Solid Edge part; units mm, degrees
sketch "Sketch1" plane through (0, 0, 0) normal (0, -1, 0) x (1, 0, 0)
  line L0 (25, -40) -> (25, 40)
  line L1 (25, 40) -> (-25, 40)
  line L2 (-25, 40) -> (-25, -40)
  line L3 (-25, -40) -> (25, -40)
  line L4 (22.5, -37.5) -> (22.5, 37.5)
  line L5 (22.5, 37.5) -> (-22.5, 37.5)
  line L6 (-22.5, 37.5) -> (-22.5, -37.5)
  line L7 (-22.5, -37.5) -> (22.5, -37.5)
extrude "Protrusion1" add sketch "Sketch1" against normal blind 35
sketch "Sketch2" plane through (0, 0, 0) normal (0, -1, 0) x (1, 0, 0)
  line L0 (22.5, 37.5) -> (-22.5, 37.5)
  line L1 (-22.5, 37.5) -> (-22.5, -37.5)
  line L2 (-22.5, -37.5) -> (22.5, -37.5)
  line L3 (22.5, -37.5) -> (22.5, 37.5)
extrude "ExtrudedProtrusion_2" add sketch "Sketch2" against normal blind 5
sketch "Sketch3" plane through (0, 0, 0) normal (0, -1, 0) x (0, 0, -1)
  circle A0 centre (-28.125, 11.25) radius 5
extrude "ExtrudedProtrusion_3" add sketch "Sketch3" along normal blind 3
pattern_linear "Pattern1" count 4 spacing 18.75 along (0, 0, -1) count 2 spacing 22.5 along (-1, 0, 0) of "ExtrudedProtrusion_3"
sketch "Sketch4" plane through (0, 5, 0) normal (0, 1, 0) x (0, 0, -1)
  line L0 (1, -9) -> (1, -22.5)
  line L1 (1, -22.5) -> (-1, -22.5)
  line L2 (-1, -22.5) -> (-1, -8.9443)
  line L3 (-1, -8.9443) -> (1, -9)
  line L4 (1, 9) -> (1, 22.5)
  line L5 (1, 22.5) -> (-1, 22.5)
  line L6 (-1, 22.5) -> (-1, 8.9443)
  line L7 (-1, 8.9443) -> (1, 9)
extrude "ExtrudedProtrusion_8" add sketch "Sketch4" along normal blind 20
sketch "Sketch5" plane through (0, 5, 19.25) normal (0, 1, 0) x (0, 0, 1)
  line L0 (-46.375, -22.5) -> (-48.375, -22.5)
  arc A0 (-48.375, -22.5) -> (-46.375, -22.5) centre (-47.375, -22.5) cw
extrude "ExtrudedProtrusion_9" add sketch "Sketch5" along normal blind 30
sketch "Sketch6" plane through (0, 5, -19.25) normal (0, 1, 0) x (1, 0, 0)
  line L0 (22.5, 8.875) -> (22.5, 9.875)
  line L1 (22.5, 7.875) -> (22.5, 8.875)
  arc A0 (22.5, 7.875) -> (22.5, 9.875) centre (22.5, 8.875) cw
  line L2 (22.5, -9.875) -> (22.5, -8.875)
  line L3 (22.5, -10.875) -> (22.5, -9.875)
  arc A1 (22.5, -10.875) -> (22.5, -8.875) centre (22.5, -9.875) cw
  line L4 (22.5, -28.625) -> (22.5, -27.625)
  line L5 (22.5, -29.625) -> (22.5, -28.625)
  arc A2 (22.5, -29.625) -> (22.5, -27.625) centre (22.5, -28.625) cw
  line L6 (22.5, -47.375) -> (22.5, -46.375)
  line L7 (22.5, -47.375) -> (22.5, -48.375)
  arc A3 (22.5, -48.375) -> (22.5, -46.375) centre (22.5, -47.375) cw
  line L8 (-22.5, -28.625) -> (-22.5, -29.625)
  line L9 (-22.5, -27.625) -> (-22.5, -28.625)
  arc A4 (-22.5, -27.625) -> (-22.5, -29.625) centre (-22.5, -28.625) cw
  line L10 (-22.5, -8.875) -> (-22.5, -10.875)
  arc A5 (-22.5, -8.875) -> (-22.5, -10.875) centre (-22.5, -9.875) cw
  line L11 (-22.5, -47.375) -> (-22.5, -48.375)
  line L12 (-22.5, -46.375) -> (-22.5, -47.375)
  arc A6 (-22.5, -46.375) -> (-22.5, -48.375) centre (-22.5, -47.375) cw
extrude "ExtrudedProtrusion_10" add sketch "Sketch6" along normal blind 30
sketch "Sketch7" plane through (0, 5, 0) normal (0, -1, 0) x (1, 0, 0)
  circle A0 centre (0, -25) radius 10
  circle A1 centre (0, -25) radius 7.5
  circle A2 centre (0, 0) radius 10
  circle A3 centre (0, 0) radius 7.5
  circle A4 centre (0, 25) radius 10
  circle A5 centre (0, 25) radius 7.5
extrude "ExtrudedProtrusion_11" add sketch "Sketch7" against normal blind 30
sketch "Sketch8" plane through (0, 5, -19.25) normal (0, 1, 0) x (1, 0, 0)
  line L0 (-12.25, 18.25) -> (-11.25, 18.25)
  line L1 (-11.25, 18.25) -> (-10.25, 18.25)
  arc A0 (-10.25, 18.25) -> (-12.25, 18.25) centre (-11.25, 18.25) cw
  line L2 (10.25, 18.25) -> (11.25, 18.25)
  line L3 (11.25, 18.25) -> (12.25, 18.25)
  arc A1 (12.25, 18.25) -> (10.25, 18.25) centre (11.25, 18.25) cw
  line L4 (11.25, -56.75) -> (12.25, -56.75)
  line L5 (11.25, -56.75) -> (10.25, -56.75)
  arc A2 (10.25, -56.75) -> (12.25, -56.75) centre (11.25, -56.75) cw
  line L6 (-10.25, -56.75) -> (-11.25, -56.75)
  line L7 (-11.25, -56.75) -> (-12.25, -56.75)
  arc A3 (-12.25, -56.75) -> (-10.25, -56.75) centre (-11.25, -56.75) cw
extrude "ExtrudedProtrusion_12" add sketch "Sketch8" along normal blind 30
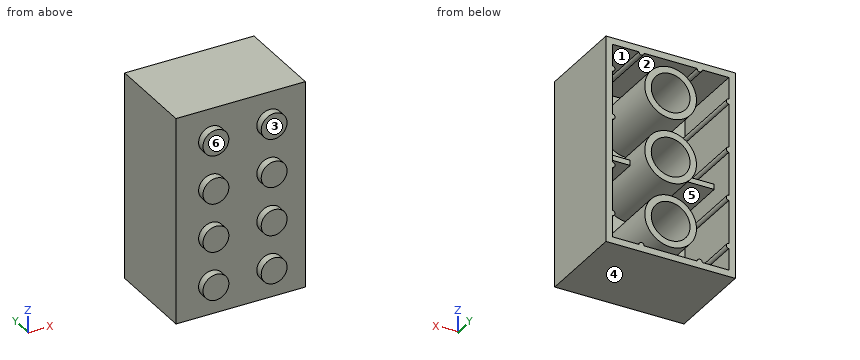
Geometry check sheet. Reference: the model listing, model coordinates, mm. Face numbers are marked on the shaded views. A direction names the side the tool comes from. Round coordinates to 2 decimals unless told otherwise and drop trailing zeros. Loops run counter-clockwise (first coordinate to the right, second up) from the corner with the lowest first, then second, coordinate; pieces in that order, holes last. Notation, with made-up numbers: (89.5, -31.5) -> (129.5, -31.5) arc R35 cw to (129.5, 7.5) -> close; hole circle Ø8 at (70, 44). An arc over 180 degrees is marked (long way). Use a Markdown table: item, result.
(1) Sectioned sample at C-C (z = 0). Enter the section's corners in (x, y), then the cut area to 3 significant figures.
Calculated:
| item | result |
|---|---|
| outline | (-25, 0) -> (25, 0) -> (25, 35) -> (22.5, 35) -> (22.5, 25) -> (10, 25) -> (10, 35) -> (7.5, 35) -> (7.5, 5) -> (-7.5, 5) -> (-7.5, 35) -> (-10, 35) -> (-10, 25) -> (-22.5, 25) -> (-22.5, 35) -> (-25, 35) -> close |
| area | 1,050 mm² |
(2) Sectioned sample at A-A (y = 26). Give the number of separate pieces and of enclosed holes in the cut face, then the cut area to 3 significant figures.
Calculated:
| item | result |
|---|---|
| separate pieces | 4 |
| enclosed holes | 4 |
| area | 1,060 mm² |
(3) Mould release check, pull along Z, two halves, no side actions. Record for the marked faces 1, 2, 3 and 4: released by +Z, released by -Z, zero draft, split by the parting line, or undercut.
Calculated:
| item | result |
|---|---|
| face 1 | undercut |
| face 2 | undercut |
| face 3 | zero draft |
| face 4 | released by -Z |
(4) Go/stop test with flat-tipped pins: P1, Ø2, axis at x = 2, z = 10, coming from the -Y side; P2, Ø0.6, axis at x = -18.5, z = 0, coming from the +Y side; P3, Ø4, axis at x = -15, z = -4, coming from the +Y side. Record where each tip stops, or that it passes through.
Calculated:
| item | result |
|---|---|
| P1 | y = 0 |
| P2 | y = 25 |
| P3 | y = 5 |
(5) Sectioned sample at B-B (x = -11.25). Enter the section's corners in (y, z) (3 decimals).
Calculated:
| item | result |
|---|---|
| outline | (-3, -33.125) -> (0, -33.125) -> (0, -40) -> (35, -40) -> (35, -36.5) -> (5, -36.5) -> (5, -1) -> (25, -1) -> (25, 1) -> (5, 1) -> (5, 36.5) -> (35, 36.5) -> (35, 40) -> (0, 40) -> (0, 33.125) -> (-3, 33.125) -> (-3, 23.125) -> (0, 23.125) -> (0, 14.375) -> (-3, 14.375) -> (-3, 4.375) -> (0, 4.375) -> (0, -4.375) -> (-3, -4.375) -> (-3, -14.375) -> (0, -14.375) -> (0, -23.125) -> (-3, -23.125) -> close |
(6) Scan lines: probe 1 along Z at (x, y) = (-17.5, 18.5); probe 2 along Z at (x, y) = (15.5, 26); probe 3 along X at (y, z) = (7, 13.5). Record each from-to range of solid material in increasing order.
Calculated:
| item | result |
|---|---|
| probe 1 | -40 to -37.5, -1 to 1, 37.5 to 40 |
| probe 2 | -40 to -37.5, 37.5 to 40 |
| probe 3 | -25 to -22.5, 22.5 to 25 |
(7) Set-up check for the marked faces 5 and 6: record each of +Z, -Z, +X, -X, +Y, -Y from which the full face is reachable in a straight line by a thin tool's end or side.
Calculated:
| item | result |
|---|---|
| face 5 | +Y |
| face 6 | +Z, -Z, +X, -X, -Y |
